from build123d import *

# Parameters (mm, degrees)
SKETCH_1_R          = 2
EXTRUDE_1_DEPTH     = 6
SKETCH_2_R          = 5.5
SKETCH_2_R_2        = 3
EXTRUDE_2_DEPTH     = 12
CUT_EXTRUDE_START   = 10
SKETCH_3_R          = 1.5
CUT_EXTRUDE_1_DEPTH = 20


with BuildPart() as part:
    # 草图1 → 凸台-拉伸1 (new body)
    with BuildSketch(Plane.XY):
        Polygon((-3.464101615, 6), (3.464101615, 6), (6.92820323, 0), (3.464101615, -6), (-3.464101615, -6), (-6.92820323, 0), align=None)
        Circle(SKETCH_1_R, mode=Mode.SUBTRACT)
    extrude(amount=EXTRUDE_1_DEPTH)

    # 草图2 → 凸台-拉伸2 (add)
    with BuildSketch(Plane(origin=(0, 0, 0), x_dir=(-1, 0, 0), z_dir=(0, 0, -1))):
        Circle(SKETCH_2_R)
        Circle(SKETCH_2_R_2, mode=Mode.SUBTRACT)
    extrude(amount=EXTRUDE_2_DEPTH)

    # 草图3 → 切除-拉伸1 (cut)
    with BuildSketch(Plane(origin=(0, 0, 0), x_dir=(1, 0, 0), z_dir=(0, 1, 0)).offset(CUT_EXTRUDE_START)):
        with Locations(Location((0, 8.269925745, 0), (0, 0, 270))):
            Circle(SKETCH_3_R)
    extrude(amount=-CUT_EXTRUDE_1_DEPTH, mode=Mode.SUBTRACT)


solid = part.part
Can you work these out from the model? Positions are in its coordinate system, mm. A direction names the side the tool comes from. Coordinates: 2 decimals unless noted, no trailing zeros. Loops run counter-clockwise (first coordinate to the right, second up) from the corner with the lowest first, then second, coordinate; pieces in that order, holes last. Notation, with made-up numbers: M -37,63.5 L 12,63.5 A21 cw 12,73.5 Z; hole C 40.5,76 d5. An arc over 180 degrees is marked long. Return JSON: item names as keys, results as strings. Group by question number.
Item 1: Thinking about a two-plate mould opening in X: for faces 3 (the flat face through (-1, -2, 0)), 4 (the flat face through (-2.4, -2.4, -12)), 5 (the cylindrical face through (-2.5, -4.9, -5.9)), which applies, released by +X, released by -X, zero draft, split by the parting line, or undercut?
Item 2: If I drill on L1, parallel to Z at x = 0, y = 4.15; L2, parallel to Y at x = 0, z = 2.1; L3, parallel to Y at x = 0, z = -4, over which ranges is the centre line in solid material (lowest first)? Write a range as from..to.
Item 3: Imagine slicing it at C-C (y = -0.5). Please give me the cut outline in (x, z), and give its area (3 significant figures).
Item 4: Imagine slicing it at A-A (x = 0). Please give me the cut outline in (y, z), and give its area (3 significant figures).
Item 5: I'm going to push flat-ended pins straight in: pin 1 Ø2.5 at (x, z) = (0, -8.27) entering from +Y; pin 2 Ø1 at (y, z) = (-1.5, -8) entering from -X; pin 3 Ø4 at (y, z) = (-1, 4) entering from +X; pin 4 Ø1 at (y, z) = (0, -8) entering from -X. Where does each tip first touch, or does it pass through?
Item 6: On a 3-axis mill with a long thin cutter (end or side, diameter ignored), from which of +Z, -Z, +X, -X, +Y, -Y can I reach the whole of each face in a straight line? I mean faces 1 (the flat face through (0, 6, 3)), 2 (the cylindrical face through (-1.61, 2.53, -5.92)). Say none if no direction works.
Item 7: Imagine slicing it at B-B (z = 4.25). Please give me the cut outline in (x, y).
Item 8: Imagine slicing it at D-D (z = -9). Please give me the cut outline in (x, y), and give its area (3 significant figures).
Verdict:
{
 "1": {"face 3": "undercut", "face 4": "zero draft", "face 5": "split by the parting line"},
 "2": {"L1": "z = -12..-9.77, -6.77..6", "L2": "y = -6..-2, 2..6", "L3": "y = -5.5..-3, 3..5.5"},
 "3": {"outline": "M -6.64,0 L -5.48,0 L -5.48,-12 L -2.96,-12 L -2.96,0 L -1.94,0 L -1.94,6 L -6.64,6 Z; M 1.94,0 L 2.96,0 L 2.96,-12 L 5.48,-12 L 5.48,0 L 6.64,0 L 6.64,6 L 1.94,6 Z", "area": "117 mm^2"},
 "4": {"outline": "M -6,0 L -5.5,0 L -5.5,-6.77 L -3,-6.77 L -3,0 L -2,0 L -2,6 L -6,6 Z; M -5.5,-12 L -3,-12 L -3,-9.77 L -5.5,-9.77 Z; M 2,0 L 3,0 L 3,-6.77 L 5.5,-6.77 L 5.5,0 L 6,0 L 6,6 L 2,6 Z; M 3,-12 L 5.5,-12 L 5.5,-9.77 L 3,-9.77 Z", "area": "93.0 mm^2"},
 "5": {"pin 1": "passes through", "pin 2": "stops at x = -5.41", "pin 3": "stops at x = 6.93", "pin 4": "stops at x = -5.5"},
 "6": {"face 1": "+Z, -Z, +X, -X, +Y", "face 2": "-Z"},
 "7": {"outline": "M -6.93,0 L -3.46,-6 L 3.46,-6 L 6.93,0 L 3.46,6 L -3.46,6 Z; hole C 0,0 d4"},
 "8": {"outline": "M -1.31,-5.34 L -1.31,-2.7 A3 cw -1.31,2.7 L -1.31,5.34 A5.5 ccw Z; M 1.31,-5.34 A5.5 ccw 1.31,5.34 L 1.31,2.7 A3 cw 1.31,-2.7 Z", "area": "53.4 mm^2"}
}
